The drawing under review shows one solid part. Ordinate dimensions are in mm from its lowest x, y, z. A direction names the side the tool comes from. Give positions to 0.01 mm unless a question says otherwise; leave off trailing zeros. Loops run counter-clockwise (first coordinate to the right, second up) from the corner with the lowest first, then second, coordinate; pieces in that order, holes last. Notation, with made-up numbers: (76.25, 23.5) - (83.25, 23.5) arc R13 ccw to (83.25, 32.5) - close; hole circle Ø8 at (69.25, 7.5). An arc over 180 degrees is marked (long way). Answer as CSV lines item,"result".
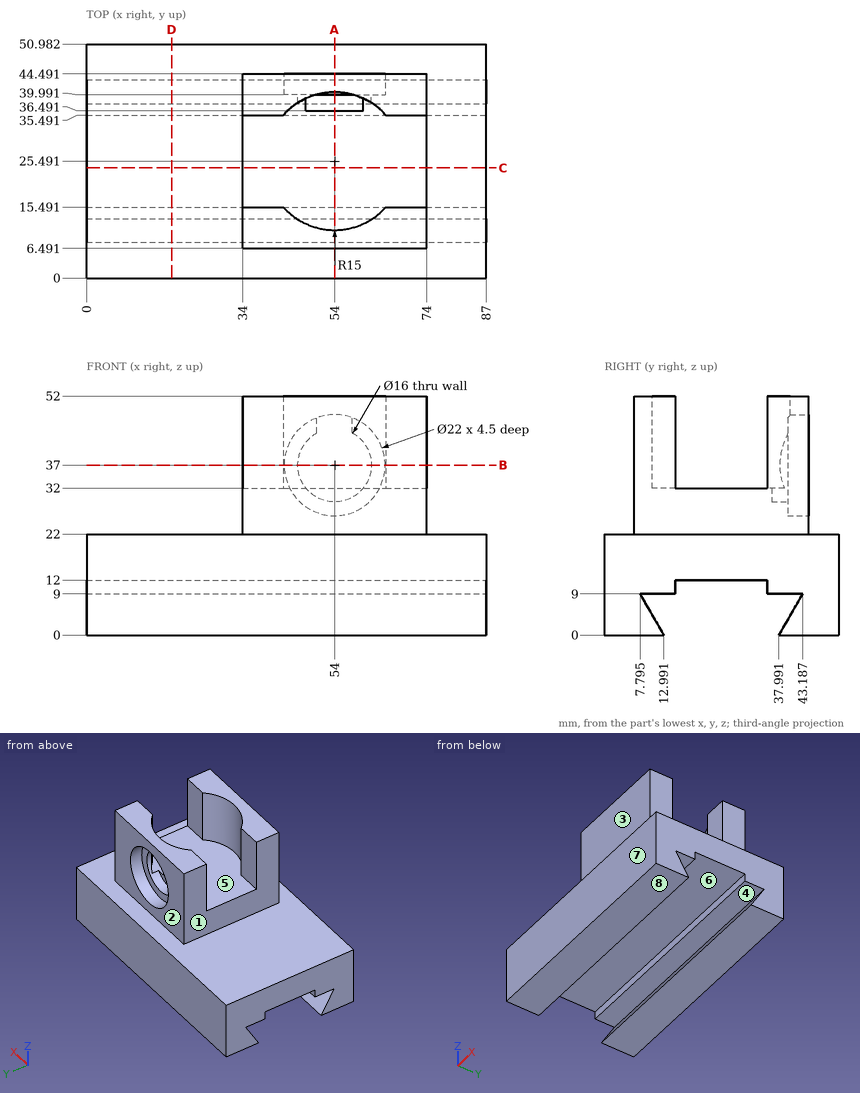
1) Wall thickness on line 1 (Y direction, x = 72, z = 10.5); line 2 (X direction, y = 43, z = 37); line 3 (Z direction, x = 71, y = 48.5): over which ranges is each line inside the solid? List them lowest first. Write a range as from..to.
From the geometry:
line 1,"y = 0..15.49, 35.49..50.98"
line 2,"x = 34..43, 65..74"
line 3,"z = 0..22"
2) Machinability: for the marked faces 1, 2, 3, 4 and 5, which of the approach directions +Z, -Z, +X, -X, +Y, -Y give a long, thin tool a straight path to every point of the face, cutting with its end or side? Answer none if there is none.
From the geometry:
face 1,"+Z, -X, +Y, -Y"
face 2,"+Z, +X, -X, +Y"
face 3,"+Z, +X, -X, -Y"
face 4,"+X, -X"
face 5,"+Z"
3) Consider section C-C on y = 24. Write out the cut boundary in (x, z).
From the geometry:
outline,"(0, 12) - (87, 12) - (87, 22) - (74, 22) - (74, 32) - (34, 32) - (34, 22) - (0, 22) - close"
4) Draft analysis for pull direction Y (two halves, no side actions). For the marked faces 6, 7 and 8, state which applies: pulls with the +Y half, pulls with the -Y half, needs draft (parallel to the pull), parting line crosses it, or undercut.
From the geometry:
face 6,"undercut"
face 7,"pulls with the -Y half"
face 8,"needs draft"
5) Consider section A-A on x = 54. Write out the cut boundary in (y, z) (3 decimals).
From the geometry:
outline,"(0, 0) - (12.991, 0) - (7.795, 9) - (15.491, 9) - (15.491, 12) - (35.491, 12) - (35.491, 9) - (43.187, 9) - (37.991, 0) - (50.982, 0) - (50.982, 22) - (44.491, 22) - (44.491, 26) - (39.991, 26) - (39.991, 29) - (36.491, 29) - (36.491, 32) - (10.491, 32) - (10.491, 52) - (6.491, 52) - (6.491, 22) - (0, 22) - close; (40.491, 48) - (44.491, 48) - (44.491, 52) - (40.491, 52) - close"
6) Consider section D-D on x = 18.5. Write out the cut boundary in (y, z) (3 decimals).
From the geometry:
outline,"(0, 0) - (12.991, 0) - (7.795, 9) - (15.491, 9) - (15.491, 12) - (35.491, 12) - (35.491, 9) - (43.187, 9) - (37.991, 0) - (50.982, 0) - (50.982, 22) - (0, 22) - close"
7) Insertion check: P1, Ø9, axis at x = 51, z = 43, coming from the +Y side; P2, Ø2, axis at x = 58, y = 28, coming from the -Z side; P3, Ø24, axis at x = 57, z = 40, coming from the -Y side; P4, Ø6, axis at y = 32, z = 35.5, coming from the -X side. Each pin has a flat end and moves straight along its axis. Give the tip position at first contact, or say it passes through.
From the geometry:
P1,"stops at y = 44.49"
P2,"stops at z = 12"
P3,"stops at y = 6.49"
P4,"passes through"
8) Consider section B-B on z = 37. Write out the cut boundary in (x, y).
From the geometry:
outline,"(34, 6.49) - (74, 6.49) - (74, 15.49) - (65.18, 15.49) arc R15 cw to (42.82, 15.49) - (34, 15.49) - close; (34, 35.49) - (42.82, 35.49) arc R15 cw to (46, 38.18) - (46, 39.99) - (43, 39.99) - (43, 44.49) - (34, 44.49) - close; (62, 38.18) arc R15 cw to (65.18, 35.49) - (74, 35.49) - (74, 44.49) - (65, 44.49) - (65, 39.99) - (62, 39.99) - close"
